```python
from build123d import *

# Parameters (mm, degrees)
SKETCH1_W           = 108.5
SKETCH1_H           = 70.5
BOSS_EXTRUDE1_DEPTH = 8
SKETCH3_W           = 102.5
SKETCH3_H           = 64.5
BOSS_EXTRUDE2_DEPTH = 1
SKETCH2_W           = 100
SKETCH2_H           = 45
CUT_EXTRUDE2_DEPTH  = 66.319407529
SKETCH4_W           = 100
SKETCH4_H           = 60.5
CUT_EXTRUDE3_DEPTH  = 3.5
SKETCH8_R           = 2.25
CUT_EXTRUDE6_DEPTH  = 66.319407529


with BuildPart() as part:
    # Sketch1 → Boss-Extrude1 (new body)
    with BuildSketch(Plane(origin=(0, 0, 0), x_dir=(1, 0, 0), z_dir=(0, 1, 0))):
        Rectangle(SKETCH1_W, SKETCH1_H)
    extrude(amount=BOSS_EXTRUDE1_DEPTH)

    # Sketch3 → Boss-Extrude2 (add)
    with BuildSketch(Plane.XZ):
        Rectangle(SKETCH3_W, SKETCH3_H)
    extrude(amount=BOSS_EXTRUDE2_DEPTH)

    # Sketch2 → Cut-Extrude2 (cut, through all)
    with BuildSketch(Plane(origin=(0, 8, 0), x_dir=(1, 0, 0), z_dir=(0, 1, 0))):
        Rectangle(SKETCH2_W, SKETCH2_H)
    extrude(amount=-CUT_EXTRUDE2_DEPTH, mode=Mode.SUBTRACT)

    # Sketch4 → Cut-Extrude3 (cut)
    with BuildSketch(Plane.XZ.offset(1)):
        Rectangle(SKETCH4_W, SKETCH4_H)
    extrude(amount=-CUT_EXTRUDE3_DEPTH, mode=Mode.SUBTRACT)

    # Sketch8 → Cut-Extrude6 (cut, through all)
    with BuildSketch(Plane(origin=(0, 8, 0), x_dir=(1, 0, 0), z_dir=(0, 1, 0))):
        with Locations(Location((-46, -27, 0), (0, 0, 270))):
            Circle(SKETCH8_R)
        with Locations(Location((46, 27, 0), (0, 0, 270))):
            Circle(SKETCH8_R)
    extrude(amount=-CUT_EXTRUDE6_DEPTH, mode=Mode.SUBTRACT)


solid = part.part
```
The listing builds one solid part. Answer for the finished solid, in the listing's coordinates (mm). A direction names the side the tool comes from. Give positions to 0.01 mm unless a question says otherwise; leave off trailing zeros. Order: outer loops, then holes, each group sorted by start corner. A loop starts at its lowest first (then second) coordinate and runs counter-clockwise, first axis right, second up. Notation, with made-up numbers: (53.25, 58.5) - (103.25, 58.5) arc R21 ccw to (103.25, 69.5) - close; hole circle Ø5 at (-27.5, 84). An arc over 180 degrees is marked (long way). Answer in a Markdown table with one row per item. Add a question column.
Q1. The part is cut by section D-D (z = -1.5). Determine the outline of the cut face in (x, y), then the cut area to 3 significant figures.
Q2. Which of the six approach directions +Z, -Z, +X, -X, +Y, -Y give full straight-line access (tool end or side, diameter ignored) to faces 5 (the flat face through (-1, 5, 22.5)), 6 (the flat face through (54.25, 4, 0)), 7 (the flat face through (-1, 1, -30.25))?
Q3. The part is cut by section A-A (x = 46). Determine the outline of the cut face in (y, z), then the cut area to 4 significant figures.
Q4. Find the intervals of material crossed by line 1 along X through (y, z) = (5.3, -27); line 2 along X through (y, z) = (3.5, 19.5); line 3 along Z through (x, y) = (24.5, 5.5), in increasing order. Write a range as [from, to].
Q5. The part is cut by section B-B (z = -27). Determine the outline of the cut face in (x, y), then the cut area to 3 significant figures.
Q6. For a pull along Z with two mould halves and no side action, classify faces 1 (the flat face through (-1, 2.5, 26)), 2 (the cylindrical face through (-44.103, 5.288, 28.21)), 3 (the flat face through (-1, 4, -35.25)), 4 (the flat face through (-1, 8, -24)) as released by +Z, released by -Z, zero draft, split by the parting line, or undercut.
Q7. Given P1, Ø7, axis at x = 46, z = -27, coming from the -Y side; P2, Ø5, axis at x = -14.5, z = -26.5, coming from the -Y side, each flat-ended and moving along its own axis, determine where each tip first touches the part or whether it passes through.
Q8. The part is cut by section C-C (x = 29). Determine the outline of the cut face in (y, z), then the cut area to 3 significant figures.
Determined:
| question | item | result |
|---|---|---|
| 1 | outline | (-54.25, 0) - (-51.25, 0) - (-51.25, -1) - (-50, -1) - (-50, 8) - (-54.25, 8) - close; (50, -1) - (51.25, -1) - (51.25, 0) - (54.25, 0) - (54.25, 8) - (50, 8) - close |
| 1 | area | 70.5 mm² |
| 2 | face 5 | +Y, -Y |
| 2 | face 6 | +Z, -Z, +X, +Y, -Y |
| 2 | face 7 | -Y |
| 3 | outline | (-1, -32.25) - (0, -32.25) - (0, -35.25) - (8, -35.25) - (8, -29.25) - (2.5, -29.25) - (2.5, -30.25) - (-1, -30.25) - close; (-1, 30.25) - (2.5, 30.25) - (2.5, 22.5) - (8, 22.5) - (8, 35.25) - (0, 35.25) - (0, 32.25) - (-1, 32.25) - close; (2.5, -24.75) - (8, -24.75) - (8, -22.5) - (2.5, -22.5) - close |
| 3 | area | 144.5 mm² |
| 4 | line 1 | x = [-54.25, 43.75], [48.25, 54.25] |
| 4 | line 2 | x = [-54.25, -50], [50, 54.25] |
| 4 | line 3 | z = [-35.25, -22.5], [22.5, 35.25] |
| 5 | outline | (-54.25, 0) - (-51.25, 0) - (-51.25, -1) - (-50, -1) - (-50, 2.5) - (43.75, 2.5) - (43.75, 8) - (-54.25, 8) - close; (48.25, 2.5) - (50, 2.5) - (50, -1) - (51.25, -1) - (51.25, 0) - (54.25, 0) - (54.25, 8) - (48.25, 8) - close |
| 5 | area | 596 mm² |
| 6 | face 1 | undercut |
| 6 | face 2 | undercut |
| 6 | face 3 | released by -Z |
| 6 | face 4 | zero draft |
| 7 | P1 | stops at y = -1 |
| 7 | P2 | stops at y = 2.5 |
| 8 | outline | (-1, -32.25) - (0, -32.25) - (0, -35.25) - (8, -35.25) - (8, -22.5) - (2.5, -22.5) - (2.5, -30.25) - (-1, -30.25) - close; (-1, 30.25) - (2.5, 30.25) - (2.5, 22.5) - (8, 22.5) - (8, 35.25) - (0, 35.25) - (0, 32.25) - (-1, 32.25) - close |
| 8 | area | 169 mm² |
